For this review, use the dimensioned drawing (mm, ordinates from the lowest corner) and the shaded views. A direction names the side the tool comes from. Round coordinates to 2 decimals unless told otherwise and drop trailing zeros. Write each loop counter-clockwise with the first axis right and the second up, starting at its lowest first coordinate (ties: lowest second). Pieces come first, ordered by that corner, then holes.
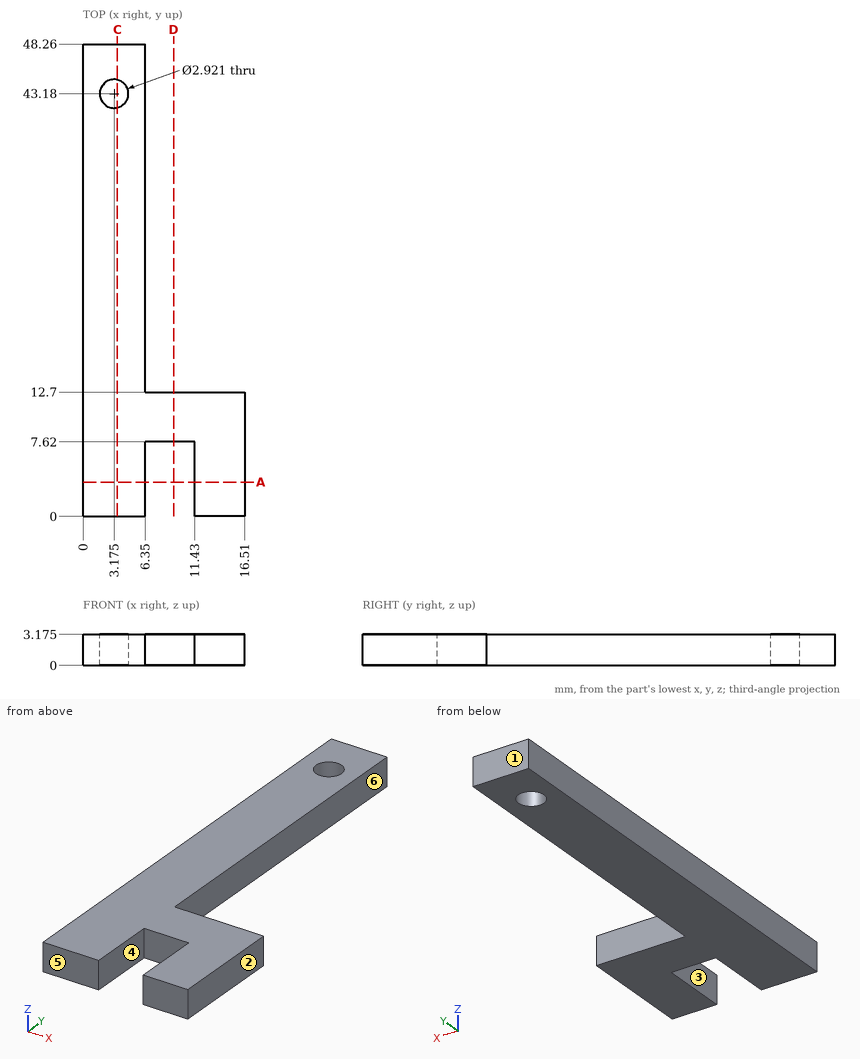
(1) For line 1 along X through (y, z) = (17, 0.7); line 2 along Y through (x, z) = (9.75, 1.4); line 3 along Y through (x, z) = (13, 1.7), list the stretches that pass through material, from the lowest coordinate up.
Geometry check:
line 1: x = 0 to 6.35
line 2: y = 7.62 to 12.7
line 3: y = 0 to 12.7
(2) For pin 1 Ø1.5 at (x, z) = (13.5, 2.5) entering from +Y; pin 2 Ø1 at (x, z) = (9, 2.5) entering from -Y; pin 3 Ø1.6 at (y, z) = (24, 1.5) entering from +X, all flat-tipped, find the tip position at first contact; note any pin that passes through.
Geometry check:
pin 1: stops at y = 12.7
pin 2: stops at y = 7.62
pin 3: stops at x = 6.35
(3) For the marked faces 4, 5 and 6, list the 3-axis set-ups (+Z, -Z, +X, -X, +Y, -Y) from which the entire face can be reached by the end or side of a thin tool; tool diameter is ignored.
Geometry check:
face 4: +Z, -Z, -Y
face 5: +Z, -Z, +X, -X, -Y
face 6: +Z, -Z, +X, +Y
(4) Mouldability with a two-part tool opening along X and no side actions: class the marked faces 1, 2 and 3 as pulls with the +X half, pulls with the -X half, needs draft (parallel to the pull), parting line crosses it, or undercut.
Geometry check:
face 1: needs draft
face 2: pulls with the +X half
face 3: undercut
(5) We need section C-C, the plane x = 3.5. Give the boundary of the cut face in (y, z) (3 decimals).
Geometry check:
outline: (0, 0) - (41.756, 0) - (41.756, 3.175) - (0, 3.175) - close; (44.604, 0) - (48.26, 0) - (48.26, 3.175) - (44.604, 3.175) - close
(6) We need section A-A, the plane y = 3.5. Give the boundary of the cut face in (x, z) (3 decimals).
Geometry check:
outline: (0, 0) - (6.35, 0) - (6.35, 3.175) - (0, 3.175) - close; (11.43, 0) - (16.51, 0) - (16.51, 3.175) - (11.43, 3.175) - close
(7) We need section D-D, the plane x = 9.25. Give the boundary of the cut face in (y, z) (3 decimals), and give its area (3 significant figures).
Geometry check:
outline: (7.62, 0) - (12.7, 0) - (12.7, 3.175) - (7.62, 3.175) - close
area: 16.1 mm2
